from build123d import *

# Parameters (mm, degrees)
SKETCH_1_W      = 100
SKETCH_1_H      = 79
SKETCH_1_R      = 1.25
EXTRUDE_1_DEPTH = 2
SKETCH_2_W      = 22.62402863
SKETCH_2_H      = 13.977148577
EXTRUDE_2_DEPTH = 3
SKETCH_3_W      = 61.437231596
SKETCH_3_H      = 32.614177876
EXTRUDE_3_DEPTH = 29
SKETCH_4_W      = 17.125360724
SKETCH_4_H      = 12.991368713
SKETCH_4_W_2    = 18.980608136
SKETCH_4_W_3    = 14.556556615
EXTRUDE_4_DEPTH = 20


with BuildPart() as part:
    # 草图1 → 凸台-拉伸1 (new body)
    with BuildSketch(Plane(origin=(0, 0, 0), x_dir=(1, 0, 0), z_dir=(0, 1, 0))):
        Rectangle(SKETCH_1_W, SKETCH_1_H)
        with Locations(Location((-46, 22.5, 0), (0, 0, 270))):
            Circle(SKETCH_1_R, mode=Mode.SUBTRACT)
        with Locations(Location((46, 22.5, 0), (0, 0, 270))):
            Circle(SKETCH_1_R, mode=Mode.SUBTRACT)
        with Locations(Location((46, -35.5, 0), (0, 0, 270))):
            Circle(SKETCH_1_R, mode=Mode.SUBTRACT)
        with Locations(Location((-46, -35.5, 0), (0, 0, 270))):
            Circle(SKETCH_1_R, mode=Mode.SUBTRACT)
    extrude(amount=EXTRUDE_1_DEPTH)

    # 草图2 → 凸台-拉伸2 (add)
    with BuildSketch(Plane.XZ):
        with Locations((-15.800196743, 15.117537052)):
            Rectangle(SKETCH_2_W, SKETCH_2_H)
    extrude(amount=EXTRUDE_2_DEPTH)

    # 草图3 → 凸台-拉伸3 (add)
    with BuildSketch(Plane(origin=(0, 2, 0), x_dir=(1, 0, 0), z_dir=(0, 1, 0))):
        with Locations((0, -23.192911062)):
            Rectangle(SKETCH_3_W, SKETCH_3_H)
    extrude(amount=EXTRUDE_3_DEPTH)

    # 草图4 → 凸台-拉伸4 (add)
    with BuildSketch(Plane(origin=(0, 2, 0), x_dir=(1, 0, 0), z_dir=(0, 1, 0))):
        with Locations((-24.938806554, 33.004315644)):
            Rectangle(SKETCH_4_W, SKETCH_4_H)
        with Locations((0.392456183, 33.004315644)):
            Rectangle(SKETCH_4_W_2, SKETCH_4_H)
        with Locations((28.435234369, 33.004315644)):
            Rectangle(SKETCH_4_W_3, SKETCH_4_H)
    extrude(amount=EXTRUDE_4_DEPTH)


solid = part.part
Check sheet for the modelled part. Datum: model origin and axes. Units: mm. A direction names the side the tool comes from. Round coordinates to 2 decimals unless told otherwise and drop trailing zeros. Order: outer loops, then holes, each group sorted by start corner. A loop starts at its lowest first (then second) coordinate and runs counter-clockwise, first axis right, second up. Notation, with made-up numbers: M 56,-16.5 L 111,-16.5 A26 ccw 111,4.5 Z; hole C 69.5,71 d11. An arc over 180 degrees is marked long. One line per item, written item: value. Start each with the question number.
1. Access from +Z, -Z, +X, -X, +Y, -Y to the whole of each face (thin tool, end or side, straight path). Record for faces 4 (the flat face through (28, 22, -33)), 5 (the flat face through (0, 16, 6.886)), 6 (the flat face through (-9.098, 12, -33)).
2. Section check A-A on y = 16. Enter the section's corners in (x, z).
3. Gauge pin test, flat ends, axial feed: P1, Ø4, axis at x = 34, z = 26, coming from the +Y side; P2, Ø10.5, axis at x = 1, z = -31.5, coming from the +Y side; P3, Ø0.9, axis at x = -17, y = -1.5, coming from the -Z side; P4, Ø1, axis at x = 36.5, y = 5.5, coming from the -Z side. Record the tip position at first contact, or that the pin passes through.
4. Scan lines: line 1 along X through (y, z) = (6.5, -32); line 2 along X through (y, z) = (0.95, -22.5); line 3 along Z through (x, y) = (6.5, 10). Record each from-to range of solid material in increasing order.
5. Section check D-D on z = 26.5. Enter the section's corners in (x, y), and give its area (3 significant figures).
6. Release check for a two-part mould opening along X. For faces 1 (the cylindrical face through (47.24, 0.99, -22.66)), 2 (the flat face through (35.714, 12, -33)), 3 (the flat face through (0, 22, -33)) record: released by +X, released by -X, zero draft, split by the parting line, or undercut.
7. Section check B-B on x = -46. Enter the section's corners in (y, z).
8. Section check C-C on z = 35.5. Enter the section's corners in (x, y), and give its area (3 significant figures).
Results found:
1. face 4: -Z, +X, -X, +Y
1. face 5: +X, -X, +Y
1. face 6: -Z, +Y
2. outline: M -33.5,-39.5 L -16.38,-39.5 L -16.38,-26.51 L -33.5,-26.51 Z; M -30.72,6.89 L 30.72,6.89 L 30.72,39.5 L -30.72,39.5 Z; M -9.1,-39.5 L 9.88,-39.5 L 9.88,-26.51 L -9.1,-26.51 Z; M 21.16,-39.5 L 35.71,-39.5 L 35.71,-26.51 L 21.16,-26.51 Z
3. P1: y = 2
3. P2: y = 22
3. P3: z = 8.13
3. P4: through
4. line 1: -33.5 to -16.38, -9.1 to 9.88, 21.16 to 35.71
4. line 2: -50 to -47.25, -44.75 to 44.75, 47.25 to 50
4. line 3: -39.5 to -26.51, 6.89 to 39.5
5. outline: M -50,0 L 50,0 L 50,2 L 30.72,2 L 30.72,31 L -30.72,31 L -30.72,2 L -50,2 Z
5. area: 1,980 mm^2
6. face 1: undercut
6. face 2: released by +X
6. face 3: zero draft
7. outline: M 0,-39.5 L 2,-39.5 L 2,-23.75 L 0,-23.75 Z; M 0,-21.25 L 2,-21.25 L 2,34.25 L 0,34.25 Z; M 0,36.75 L 2,36.75 L 2,39.5 L 0,39.5 Z
8. outline: M -50,0 L -47.25,0 L -47.25,2 L -50,2 Z; M -44.75,0 L 44.75,0 L 44.75,2 L 30.72,2 L 30.72,31 L -30.72,31 L -30.72,2 L -44.75,2 Z; M 47.25,0 L 50,0 L 50,2 L 47.25,2 Z
8. area: 1,970 mm^2
